Check sheet for the modelled part. Datum: model origin and axes. Units: mm. Face numbers are marked on the shaded views. A direction names the side the tool comes from. Give positions to 0.01 mm unless a question says otherwise; leave off trailing zeros. Order: outer loops, then holes, each group sorted by start corner. A loop starts at its lowest first (then second) coordinate and runs counter-clockwise, first axis right, second up.
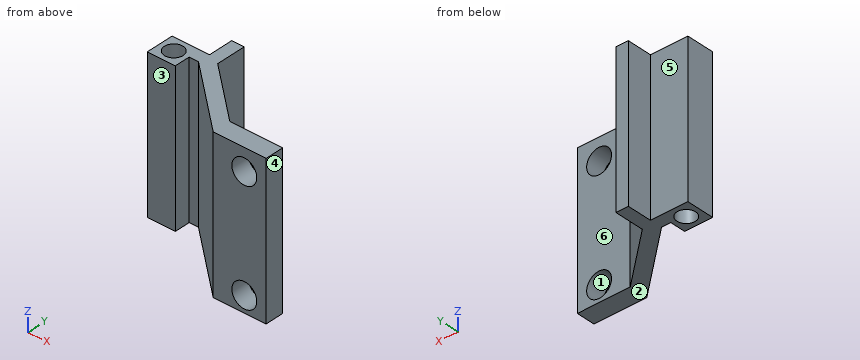
Autodesk Inventor part; units mm, degrees
ref_plane "YZ Plane" through (0, 0, 0) normal (1, 0, 0) x (0, 1, 0)
ref_plane "XZ Plane" through (0, 0, 0) normal (0, 1, 0) x (-1, 0, 0)
ref_plane "XY Plane" through (0, 0, 0) normal (0, 0, 1) x (1, 0, 0)
sketch "Sketch1" plane through (0, 0, 0) normal (0, 1, 0) x (-1, 0, 0)
  line L0 (0, 0) -> (0, -18)
  circle A0 centre (0, 0) radius 2
  circle A1 centre (0, -18) radius 2
  line L1 (0, -18) -> (5, -18)
  line L2 (5, -18) -> (5, -20.5922)
  line L3 (5, -20.5922) -> (0, -20.5922)
  line L4 (0, -20.5922) -> (0, -18)
  line L5 (0, 0) -> (-3.5, 0)
  line L6 (-3.5, 0) -> (-3.5, 3.5)
  line L7 (-3.5, 3.5) -> (0, 3.5)
  line L8 (0, 3.5) -> (0, 0)
  line L9 (-3.5, 3.5) -> (5, 3.5)
  line L10 (5, 3.5) -> (5, -20.5922)
  line L11 (5, -20.5922) -> (-3.5, -20.5922)
  line L12 (-3.5, -20.5922) -> (-3.5, 3.5)
  dimension "d0" = 18
  dimension "d1" = 4
  dimension "d2" = 4
  dimension "d3" = 5
  dimension "d4" = 3.5
  dimension "d5" = 3.5
extrude "Extrusion1" add sketch "Sketch1" along normal blind 3 contours A0 L8 L9 L10 L1 A1 L0 | L0 A1 L4 L11 L12 L5 A0 | L5 L6 L7 L8 A0 | L1 L2 L3 L4 A1
sketch "Sketch2" plane through (-5, 0, 3.5) normal (0, 0, 1) x (1, 0, 0)
  line L0 (0, 3) -> (4.25, 3)
  line L1 (0, 3) -> (8.5, 3)
  line L2 (4.25, 3) -> (-96.75, 3)
  line L3 (-46.25, 3) -> (-11.25, 3)
  line L4 (-11.25, 3) -> (-11.25, 13)
  line L5 (-11.25, 13) -> (0, 3)
  line L6 (-11.25, 13) -> (-11.25, 10)
  line L7 (0, 0) -> (0, 3)
  line L8 (-11.25, 10) -> (0, 0)
  line L9 (-11.25, 10) -> (-17.25, 10)
  line L10 (-17.25, 10) -> (-17.25, 12)
  line L11 (-17.25, 12) -> (-11.25, 12)
  line L12 (-11.25, 12) -> (-11.25, 10)
  line L13 (-11.25, 10) -> (-9.25, 10)
  line L14 (-9.25, 10) -> (-9.25, 16)
  line L15 (-9.25, 16) -> (-11.25, 16)
  line L16 (-11.25, 16) -> (-11.25, 10)
  line L17 (-17.25, 10) -> (-12.75, 10)
  line L18 (-12.75, 10) -> (-12.75, 7.5)
  line L19 (-12.75, 7.5) -> (-17.25, 7.5)
  line L20 (-17.25, 7.5) -> (-17.25, 10)
  line L21 (-15, 10) -> (-15, 9.75)
  circle A0 centre (-15, 9.75) radius 1.5
  point P0 (5, 0)
  point P1 (-11.25, 12)
  point P2 (-11.25, 13)
  point P3 (-9.25, 11.2222)
  dimension "d8" = 101
  dimension "d9" = 35
  dimension "d10" = 10
  dimension "d11" = 3
  dimension "d12" = 6
  dimension "d13" = 2
  dimension "d17" = 2
  dimension "d18" = 6
  dimension "d25" = 4.5
  dimension "d26" = 2.5
  dimension "d27" = 0.25
  dimension "d28" = 3
extrude "Extrusion2" add sketch "Sketch2" against normal up to surface (24.0922 mm away) contours L7 L8 L2 | L2 L8 L13 L14 L5 | L14 L13 L4 L5 | L5 L16 L15 L14 | L9 A0 L10 L11 L4 | L18 L19 L20 L9 A0
properties part number "suport3_pcb_temp"
(1) Cross-section at A-A on x = 0. Enter the section's corners in (y, z).
Response values:
outline: (0, -20.59) - (3, -20.59) - (3, -20) - (0, -20) - close; (0, -16) - (3, -16) - (3, -2) - (0, -2) - close; (0, 2) - (3, 2) - (3, 3.5) - (0, 3.5) - close
(2) Release check for a two-part mould opening along Z. For the marked faces 1, 2 and 3 record: released by +Z, released by -Z, zero draft, split by the parting line, or undercut.
Response values:
face 1: undercut
face 2: released by -Z
face 3: zero draft
(3) Cross-section at C-C on z = -6.5. Enter the section's corners in (x, y), then the cut area to 3 significant figures.
Response values:
outline: (-22.25, 7.5) - (-17.75, 7.5) - (-17.75, 10) - (-16.25, 10) - (-5, 0) - (3.5, 0) - (3.5, 3) - (-5, 3) - (-14.25, 11.22) - (-14.25, 16) - (-16.25, 16) - (-16.25, 12) - (-22.25, 12) - close; hole circle Ø3 at (-20, 9.75)
area: 83.2 mm2
(4) Set-up check for the marked faces 4, 5 and 6: record each of +Z, -Z, +X, -X, +Y, -Y from which the full face is reachable in a straight line by a thin tool's end or side.
Response values:
face 4: +Z, -Z, +X, +Y, -Y
face 5: +Z, -Z, -X, +Y
face 6: +Z, -Z, +X, +Y
(5) Material ranges on L1, parallel to Z at x = 0, y = 1.05; L2, parallel to Y at x = -20, z = -8.75; L3, parallel to X at y = 8.5, z = -12, recorded low to high.
Response values:
L1: z = -20.59 to -20, -16 to -2, 2 to 3.5
L2: y = 7.5 to 8.25, 11.25 to 12
L3: x = -22.25 to -20.83, -19.17 to -17.75, -14.56 to -11.19
(6) Cross-section at B-B on z = -18. Enter the section's corners in (x, y).
Response values:
outline: (-22.25, 7.5) - (-17.75, 7.5) - (-17.75, 10) - (-16.25, 10) - (-5, 0) - (-2, 0) - (-2, 3) - (-5, 3) - (-14.25, 11.22) - (-14.25, 16) - (-16.25, 16) - (-16.25, 12) - (-22.25, 12) - close; (2, 0) - (3.5, 0) - (3.5, 3) - (2, 3) - close; hole circle Ø3 at (-20, 9.75)
(7) Cross-section at D-D on x = -20. Enter the section's corners in (y, z).
Response values:
outline: (7.5, -20.59) - (8.25, -20.59) - (8.25, 3.5) - (7.5, 3.5) - close; (11.25, -20.59) - (12, -20.59) - (12, 3.5) - (11.25, 3.5) - close
(8) Gauge pin test, flat ends, axial feed: pin 1 Ø8 at (x, z) = (-17, -10) entering from -Y; pin 2 Ø6 at (x, z) = (-9.5, -7.5) entering from -Y; pin 3 Ø2.5 at (y, z) = (13.5, -12) entering from +X. Record the tip position at first contact, or that the pin passes through.
Response values:
pin 1: stops at y = 7.11
pin 2: stops at y = 1.33
pin 3: stops at x = -14.25
